```python
from build123d import *

# Parameters (mm, degrees)
EXTRUDE1_DEPTH    = 56.3372
HOLE2_D           = 23.876
HOLE2_DEPTH       = 6.35
SKETCH6_W         = 9.5123
SKETCH6_H         = 0.9398
HOLE3_D           = 6.7818
HOLE3_DEPTH       = 12.7
CIRPATTERN1_COUNT = 2
LPATTERN1_COUNT   = 2
LPATTERN1_PITCH   = 25.4
EXTRUDE2_DEPTH    = 6.78


with BuildPart() as part:
    # Sketch1 → Extrude1 (new body)
    with BuildSketch(Plane.XY.offset(56.3372)):
        with BuildLine():
            Line((23.233094839, 8.501241812), (12.7, 37.2872))
            Line((12.7, 37.2872), (-12.7, 37.2872))
            Line((-12.7, 37.2872), (-23.233094839, 8.501241812))
            ThreePointArc((-23.233094839, 8.501241812), (0, -24.7396), (23.233094839, 8.501241812))
        make_face()
    extrude(amount=-EXTRUDE1_DEPTH)

    # Hole2
    with Locations(Plane(origin=(0, 0, 0), x_dir=(-1, 0, 0), z_dir=(0, 0, -1))):
        with Locations((0, 0)):
            Hole(HOLE2_D / 2, depth=HOLE2_DEPTH)

    # Sketch7 → Revolve2 (revolve)
    with BuildSketch(Plane.XZ):
        Polygon((9.5123, 68.1228), (0, 68.1228), (0, 56.3372), (23.8125, 56.3372), (23.8125, 62.6872), (9.5123, 62.6872), align=None)
    revolve(axis=Axis((0, 0, 0), (0, 0, 1)))

    # Sketch6 → Revolve1 (revolve)
    with BuildSketch(Plane.XZ):
        with Locations((4.75615, 5.8801)):
            Rectangle(SKETCH6_W, SKETCH6_H)
    revolve(axis=Axis((0, 0, 0), (0, 0, 1)))

    # Sketch9 → Cut-Revolve1 (revolve, cut)
    with BuildSketch(Plane.XY.offset(18.2372), mode=Mode.PRIVATE) as cut_revolve1_sk:
        Polygon((-4.4196, 21.7932), (0, 21.7932), (0, 37.2872), (-8.255, 37.2872), (-8.255, 37.0332), (-5.0165, 37.0332), (-5.0165, 37.0078), (-4.4196, 36.4109), align=None)
    cut_revolve1 = revolve(cut_revolve1_sk.sketch.rotate(Axis((0, 37.2872, 18.2372), (0, -1, 0)), 90), axis=Axis((0, 37.2872, 18.2372), (0, -1, 0)), mode=Mode.SUBTRACT)  # turned: the seam where the file's is

    # Hole3
    with Locations(Plane(origin=(0, 0, 0), x_dir=(-1, 0, 0), z_dir=(0, 0, -1))):
        with Locations((-18.0086, 0)):
            hole3 = Hole(HOLE3_D / 2, depth=HOLE3_DEPTH)

    # CirPattern1: Hole3 ×2 about axis
    cirpattern1_axis = Axis((0, 0, 0), (0, 0, 1))
    for i in range(1, CIRPATTERN1_COUNT):
        add(hole3.rotate(cirpattern1_axis, i * 360 / CIRPATTERN1_COUNT), mode=Mode.SUBTRACT)

    # Sketch15 → Hole5 (revolve, cut)
    with BuildSketch(Plane(origin=(0, 0, 5.4102), x_dir=(0, 1, 0), z_dir=(1, 0, 0))):
        Polygon((0, 0), (0, 62.7126), (5.1308, 62.7126), (5.1308, 48.721128092), (6.7437, 47.752), (6.7437, 0), align=None)
    revolve(axis=Axis((0, 0, -0.719823899), (0, 0, 1)), mode=Mode.SUBTRACT)

    # LPattern1: Cut-Revolve1 ×2
    with Locations(*[(0, 0, i * LPATTERN1_PITCH) for i in range(1, LPATTERN1_COUNT)]):
        add(cut_revolve1, mode=Mode.SUBTRACT)

    # Sketch17 → Extrude2 (add)
    with BuildSketch(Plane(origin=(0, 37.0332, 0), x_dir=(1, 0, 0), z_dir=(0, 1, 0))):
        Polygon((8.065583261, -43.6372), (4.03279163, -36.6522), (-4.03279163, -36.6522), (-8.065583261, -43.6372), (-4.03279163, -50.6222), (4.03279163, -50.6222), align=None)
    extrude(amount=EXTRUDE2_DEPTH)

    # Sketch18 → Cut-Revolve2 (revolve, cut)
    with BuildSketch(Plane(origin=(0, 0, 0), x_dir=(0, 0, -1), z_dir=(1, 0, 0)), mode=Mode.PRIVATE) as cut_revolve2_sk:
        with BuildLine():
            Line((-49.0982, 43.8132), (-49.0982, 46.8132))
            Line((-49.0982, 46.8132), (-53.6222, 46.8132))
            Line((-53.6222, 46.8132), (-53.6222, 42.2892))
            Line((-53.6222, 42.2892), (-50.6222, 42.2892))
            ThreePointArc((-50.6222, 42.2892), (-50.175830735, 43.366830735), (-49.0982, 43.8132))
        make_face()
    revolve(cut_revolve2_sk.sketch.rotate(Axis((0, 21.7932, 43.6372), (0, 1, 0)), 180), axis=Axis((0, 21.7932, 43.6372), (0, 1, 0)), mode=Mode.SUBTRACT)  # turned: the seam where the file's is


solid = part.part
```
The model under review builds one solid part; all positions refer to its coordinate system, in mm. A direction names the side the tool comes from. Round coordinates to 2 decimals unless told otherwise and drop trailing zeros. Loops run counter-clockwise (first coordinate to the right, second up) from the corner with the lowest first, then second, coordinate; pieces in that order, holes last. Notation, with made-up numbers: (22.25, 21) -> (55.25, 21) arc R35 cw to (55.25, 57) -> close; hole circle Ø8 at (54.25, 84.5). An arc over 180 degrees is marked (long way). Answer as a JSON object with one key per item and string values. Group by question number.
1) For pin 1 Ø0.6 at (x, z) = (-7, 42.5) entering from +Y; pin 2 Ø4 at (x, z) = (11.5, 50) entering from +Y; pin 3 Ø1 at (x, z) = (-2.5, 49.5) entering from +Y, all flat-tipped, find the tip position at first contact; note any pin that passes through.
2) For faces 1 (the face through (4, 42.289, 50)), 2 (the face through (-18, 0, 12.7)), 3 (the face through (0, 21.793, 44)), list the 3-axis set-ups (+Z, -Z, +X, -X, +Y, -Y) from which the entire face can be reached by the end or side of a thin tool; tool diameter is ignored.
3) We need section B-B on y = 34.5. Write out the cut boundary in (x, z).
4) We need section A-A on z = 28.5. Write out the cut boundary in (x, y), then the cut area to 3 significant figures.
5) Mouldability with a two-part tool opening along Y and no side actions: class faces 4 (the face through (-5.087, -0.668, 61.029)), 5 (the face through (-14.62, -0.15, 6.44)), 6 (the face through (6.077, 39.624, 40.194)), 7 (the face through (-7, 37.033, 41)) as released by +Y, released by -Y, zero draft, split by the parting line, or undercut.
6) For line 1 (X direction, y = 4, z = 11.5); line 2 (Z direction, x = -8, y = 3.5); line 3 (Z direction, x = 12.5, y = -6), list the stretches that pass through material, from the lowest coordinate up. Write a range as [from, to].
7) We need section D-D on x = 18. Write out the cut boundary in (y, z), then the cut area to 3 significant figures.
8) We need section C-C on y = 18. Write out the cut boundary in (x, z).
Result set:
{
 "1": {"pin 1": "y = 43.03", "pin 2": "y = 37.29", "pin 3": "y = 43.76"},
 "2": {"face 1": "+Z, +X, +Y", "face 2": "-Z", "face 3": "none"},
 "3": {"outline": "(-13.72, 0) -> (13.72, 0) -> (13.72, 56.34) -> (-13.72, 56.34) -> close; hole circle Ø8.84 at (0, 18.24); hole circle Ø8.84 at (0, 43.64)"},
 "4": {"outline": "(-23.23, 8.5) arc R24.74 ccw (long way) to (23.23, 8.5) -> (12.7, 37.29) -> (-12.7, 37.29) -> close; hole circle Ø13.49 at (0, 0)", "area": "2,270 mm²"},
 "5": {"face 4": "undercut", "face 5": "undercut", "face 6": "zero draft", "face 7": "released by +Y"},
 "6": {"line 1": "[-24.41, -5.43], [5.43, 24.41]", "line 2": "[5.41, 68.12]", "line 3": "[0, 62.69]"},
 "7": {"outline": "(-16.97, 0) -> (-3.39, 0) -> (-3.39, 12.7) -> (3.39, 12.7) -> (3.39, 0) -> (22.8, 0) -> (22.8, 56.34) -> (15.59, 56.34) -> (15.59, 62.69) -> (-15.59, 62.69) -> (-15.59, 56.34) -> (-16.97, 56.34) -> close", "area": "2,350 mm²"},
 "8": {"outline": "(-19.76, 0) -> (19.76, 0) -> (19.76, 56.34) -> (15.59, 56.34) -> (15.59, 62.69) -> (-15.59, 62.69) -> (-15.59, 56.34) -> (-19.76, 56.34) -> close"}
}
